Study the drawing (mm; zero at the part's minimum x, y, z) and answer. A direction names the side the tool comes from. Coordinates: 2 decimals unless noted, no trailing zeros. Order: outer loops, then holes, each group sorted by start corner. A loop starts at its lowest first (then second) coordinate and runs counter-clockwise, first axis right, second up.
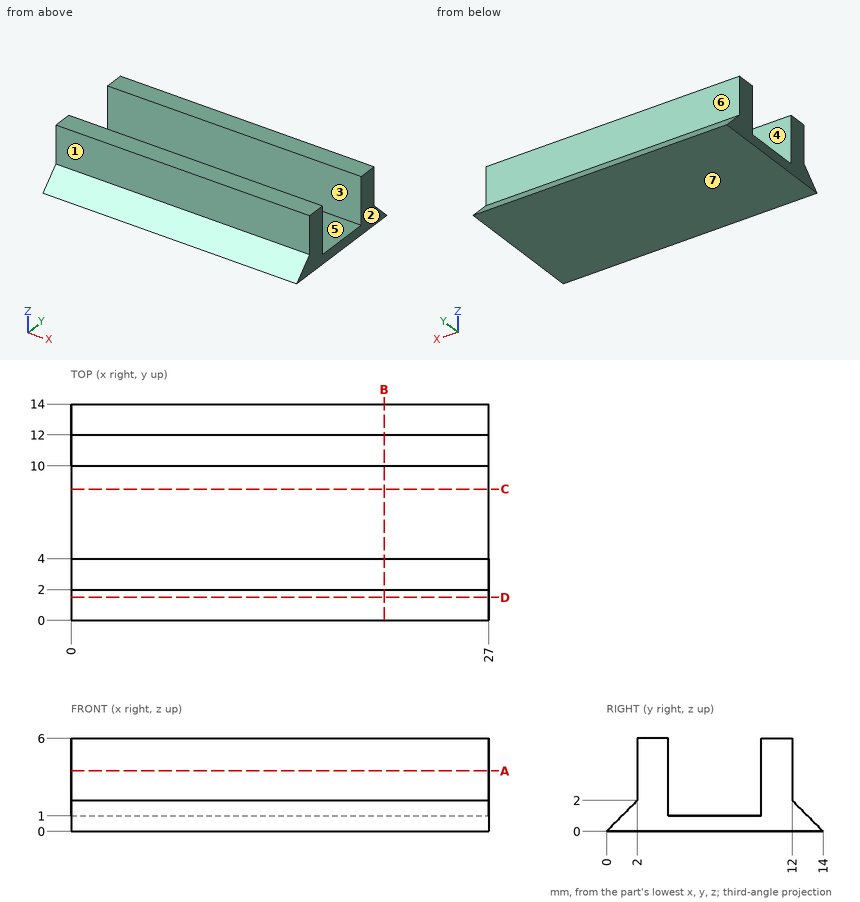
(1) Find section A-A (z = 3.9). Write down the section's boundary in (x, y).
(2) Find section B-B (x = 20.25). Write down the section's boundary in (y, z).
(3) Consider line 1 (Y direction, x = 11, z = 4.8); line 2 (Z direction, x = 11, y = 8.5); line 3 (Y direction, x = 4.75, z = 1.15). Determine where each line is inside the solid, lowest interval first.
(4) Find section C-C (y = 8.5). Write down the section's boundary in (x, z).
(5) Find section D-D (y = 1.5). Write down the section's boundary in (x, z), and give its area (3 significant figures).
(6) For the marked faces 1, 2 and 3, determine the directions among +Z, -Z, +X, -X, +Y, -Y from which every point of the face is accessible in a straight line to the end or side of a thin tool.
(7) Each of these flat-tipped pins is pushed along its axis until it touches: pin 1 Ø2.5 at (x, z) = (11, 4.5) entering from -Y; pin 2 Ø1.5 at (x, z) = (14, 3) entering from +Y; pin 3 Ø3 at (x, y) = (15, 8) entering from +Z. Where does it stop, or does it pass through?
(8) The mould has two halves that part along Y. Classify the marked faces 4, 5, 6 and 7: released by +Y, released by -Y, zero draft, split by the parting line, or undercut.
Findings below:
1. outline: (0, 2) - (27, 2) - (27, 4) - (0, 4) - close; (0, 10) - (27, 10) - (27, 12) - (0, 12) - close
2. outline: (0, 0) - (14, 0) - (12, 2) - (12, 6) - (10, 6) - (10, 1) - (4, 1) - (4, 6) - (2, 6) - (2, 2) - close
3. line 1: y = 2 to 4, 10 to 12
3. line 2: z = 0 to 1
3. line 3: y = 1.15 to 4, 10 to 12.85
4. outline: (0, 0) - (27, 0) - (27, 1) - (0, 1) - close
5. outline: (0, 0) - (27, 0) - (27, 1.5) - (0, 1.5) - close
5. area: 40.5 mm2
6. face 1: +Z, +X, -X, -Y
6. face 2: +Z, -Z, +X, +Y, -Y
6. face 3: +Z, +X, -X
7. pin 1: stops at y = 2
7. pin 2: stops at y = 12
7. pin 3: stops at z = 1
8. face 4: undercut
8. face 5: undercut
8. face 6: released by +Y
8. face 7: zero draft
